Verification items for the finished model (mm, model axes). A direction names the side the tool comes from. Round coordinates to 2 decimals unless told otherwise and drop trailing zeros. Write each loop counter-clockwise with the first axis right and the second up, starting at its lowest first coordinate (ties: lowest second). Pieces come first, ordered by that corner, then holes. Notation, with made-up numbers: M 47.5,0.5 L 88.5,0.5 A15 ccw 88.5,8.5 Z; hole C -0.5,3.5 d4. An arc over 180 degrees is marked long. One line per question, with ' | ' between items.
from build123d import *

# Parameters (mm, degrees)
F0_W     = 88.9
F0_H     = 88.9
F1_DEPTH = 25.4
F2_R     = 31.75
F3_DEPTH = 38.1
F4_R     = 5.08


with BuildPart() as f1:
    # F0 (on Top) → F1 (new body)
    with BuildSketch(Plane.XY):
        Rectangle(F0_W, F0_H)
    extrude(amount=F1_DEPTH)

    # F2 (on face) → F3 (join)
    with BuildSketch(Plane.XY.offset(25.4)):
        Circle(F2_R)
    extrude(amount=F3_DEPTH)

    # F4
    f4_edges = [f1.edges().sort_by_distance(p)[0] for p in [
        (-31.75, 0, 63.5),
        (-31.75, 0, 25.4),
        (44.45, 0, 25.4),
        (0, -44.45, 25.4),
        (-44.45, 0, 25.4),
        (0, 44.45, 25.4),
    ]]
    fillet(f4_edges, radius=F4_R)


solid = f1.part
1. Section check C-C, the plane z = 45. Record the cut outline in (x, y), then the cut area to 3 significant figures.
Results:
outline: C 0,0 d63.5 | area: 3,170 mm2
2. Thickness scan on line 1 (Z direction, x = 4, y = 37); line 2 (Y direction, x = -0.5, z = 29); line 3 (Y direction, x = 16.5, z = 57). Record the ranges inside material, lowest first.
Results:
line 1: z = 0 to 25.4 | line 2: y = -31.97 to 31.97 | line 3: y = -27.13 to 27.13
3. Section check A-A, the plane y = 0. Record the cut outline in (x, z), then the cut area to 3 significant figures.
Results:
outline: M -44.45,0 L 44.45,0 L 44.45,20.32 A5.08 ccw 39.37,25.4 L 36.83,25.4 A5.08 cw 31.75,30.48 L 31.75,58.42 A5.08 ccw 26.67,63.5 L -26.67,63.5 A5.08 ccw -31.75,58.42 L -31.75,30.48 A5.08 cw -36.83,25.4 L -39.37,25.4 A5.08 ccw -44.45,20.32 Z | area: 4,670 mm2
4. Tool access check on faces 1 (the face through (0.622, -43.001, 23.872)), 2 (the face through (-6.883, -30.995, 44.254)). Record the directions out of +Z, -Z, +X, -X, +Y, -Y that give a thin tool (end or side, any length) a straight path to the whole face; none if there is none.
Results:
face 1: +Z, +X, -X, -Y | face 2: +Z
5. Go/stop test with flat-tipped pins: P1, Ø4, axis at x = -27.5, z = 52.5, coming from the -Y side; P2, Ø6, axis at x = 30, z = 33, coming from the +Y side; P3, Ø2, axis at y = -15, z = 55, coming from the -X side. Record where each tip stops, or that it passes through.
Results:
P1: stops at y = -18.92 | P2: stops at y = 16.71 | P3: stops at x = -28.5
